Can you work these out from the drawing? Everything is in mm from the part's minimum corner. Coordinates: 2 decimals unless noted, no trailing zeros. Order: outer loops, then holes, each group sorted by start corner. A loop starts at its lowest first (then second) coordinate and runs counter-clockwise, first axis right, second up. Notation, with made-up numbers: (32, 37) - (81, 37) arc R23 cw to (81, 45) - close; hole circle Ø11 at (-19.5, 53.5). An arc over 180 degrees is marked (long way). One line per item, written item: value.
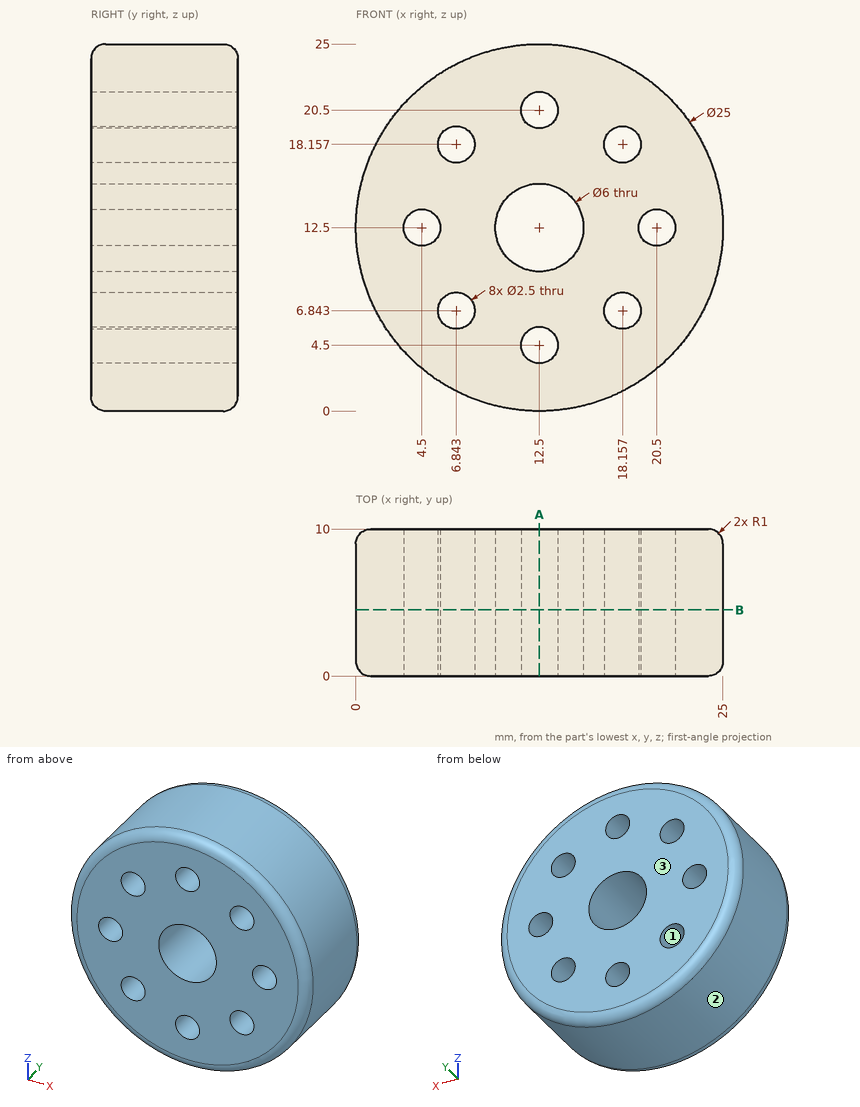
Item 1: I want a section at B-B on y = 4.5. Give the number of separate pieces and of enclosed holes in the cut face, then the cut area to 3 significant figures.
Conclusion:
separate pieces: 1
enclosed holes: 9
area: 423 mm²
Item 2: I want a section at A-A on x = 12.5. Please give me the cut outline in (y, z), then the cut area to 3 significant figures.
Conclusion:
outline: (0, 1) arc R1 ccw to (1, 0) - (9, 0) arc R1 ccw to (10, 1) - (10, 3.25) - (0, 3.25) - close; (0, 5.75) - (10, 5.75) - (10, 9.5) - (0, 9.5) - close; (0, 15.5) - (10, 15.5) - (10, 19.25) - (0, 19.25) - close; (0, 21.75) - (10, 21.75) - (10, 24) arc R1 ccw to (9, 25) - (1, 25) arc R1 ccw to (0, 24) - close
area: 139 mm²
Item 3: I'm going to push flat-ended pins straight in: pin 1 Ø5 at (y, z) = (7, 6.5) entering from -X; pin 2 Ø6 at (x, y) = (7.5, 5) entering from -Z; pin 3 Ø1.5 at (x, y) = (15, 9) entering from -Z; pin 4 Ø2 at (x, z) = (18.16, 6.84) entering from +Y. Where does each tip first touch, or does it pass through?
Conclusion:
pin 1: x = 0.5
pin 2: z = 0.16
pin 3: z = 0.12
pin 4: through
Item 4: Thinking about a two-plate mould opening in X: for the marked faces 1, 2 and 3, which applies, pulls with the +X half, pulls with the -X half, needs draft (parallel to the pull), parting line crosses it, or undercut?
Conclusion:
face 1: undercut
face 2: parting line crosses it
face 3: needs draft
Item 5: If I drill on probe 1 along X at (y, z) = (2.75, 12.5); probe 2 along X at (y, z) = (8.5, 13.5); probe 3 along X at (y, z) = (0.75, 18), over which ranges is the centre line in solid material (lowest first)?
Conclusion:
probe 1: 0 to 3.25, 5.75 to 9.5, 15.5 to 19.25, 21.75 to 25
probe 2: 0.04 to 3.75, 5.25 to 9.67, 15.33 to 19.75, 21.25 to 24.96
probe 3: 1.31 to 5.6, 8.08 to 16.92, 19.4 to 23.69
